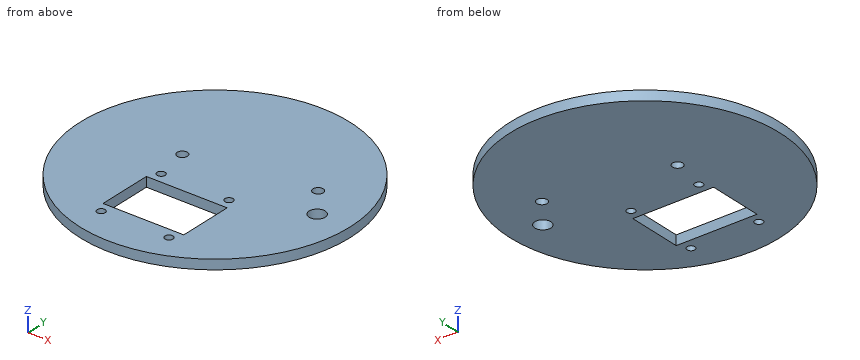
Autodesk Inventor part; units mm, degrees
ref_plane "YZ Plane" through (0, 0, 0) normal (1, 0, 0) x (0, 1, 0)
ref_plane "XZ Plane" through (0, 0, 0) normal (0, 1, 0) x (-1, 0, 0)
ref_plane "XY Plane" through (0, 0, 0) normal (0, 0, 1) x (1, 0, 0)
sketch "Эскиз3" plane through (0, 0, 0) normal (0, 0, 1) x (1, 0, 0)
  circle A0 centre (0, 0) radius 41.5
  line L0 (12.5, -11.0597) -> (-12.5, -11.0597)
  line L1 (-12.5, -11.0597) -> (-12.5, -28.0597)
  line L2 (-12.5, -11.0597) -> (12.5, -11.0597)
  line L3 (12.5, -11.0597) -> (12.5, -28.0597)
  line L4 (12.5, -28.0597) -> (-12.5, -28.0597)
  line L5 (-12.5, -28.0597) -> (-12.5, -11.0597)
  dimension "d9" = 83
  dimension "d10" = 25
  dimension "d11" = 17
  dimension "d13" = 25
  dimension "d14" = 17
  dimension "d15" = 12.5
extrude "Выдавливание3" add sketch "Эскиз3" along normal blind 3
sketch "Эскиз4" plane through (0, 0, 3) normal (0, 0, 1) x (1, 0, 0)
  arc A0 (5.7629, -8.6636) -> (-4.709, -8.7124) centre (0.4132, 15.7598) ccw
  circle A1 centre (0.4132, 15.7598) radius 1.5338
  point P0 (0, 0)
extrude "Выдавливание4" cut sketch "Эскиз4" against normal blind 3
sketch "Эскиз5" plane through (0, 0, 3) normal (0, 0, 1) x (1, 0, 0)
  line L0 (-51.8221, -46.0116) -> (-45.155, -49.3714)
  circle A0 centre (31.5626, 0.0623) radius 2.5
  point P0 (0, 0)
  dimension "d20" = 5
extrude "Выдавливание5" cut sketch "Эскиз5" against normal blind 3
sketch "Эскиз6" plane through (0, 0, 3) normal (0, 0, 1) x (1, 0, 0)
  circle A0 centre (0.4132, 15.7598) radius 1.5338
  point P0 (0, 0)
extrude "Выдавливание6" add sketch "Эскиз6" against normal blind 3
sketch "Эскиз7" plane through (0, 0, 3) normal (0, 0, 1) x (1, 0, 0)
  circle A0 centre (10.5, -7.8097) radius 1.25
  circle A1 centre (-10.5, -7.8097) radius 1.25
  circle A2 centre (-10.5, -31.3097) radius 1.25
  circle A3 centre (10.5, -31.3097) radius 1.25
  point P0 (0, 0)
extrude "Выдавливание7" cut sketch "Эскиз7" against normal blind 3
sketch "Эскиз13" plane through (0, 0, 3) normal (0, 0, 1) x (1, 0, 0)
  circle A0 centre (0, 0) radius 41.5
  circle A1 centre (0, 0) radius 41.7806
  point P0 (-26.934, 31.9403)
extrude "Выдавливание12" add sketch "Эскиз13" against normal blind 3
sketch "Эскиз14" plane through (0, 0, 0) normal (0, 0, -1) x (-1, 0, 0)
  circle A0 centre (-24.602, 9.2303) radius 1.6
  circle A1 centre (12.434, 2.9402) radius 1.6
  point P0 (0, 0)
extrude "Выдавливание13" cut sketch "Эскиз14" against normal blind 3
equation "\"d13\" = d10"
equation "\"d14\" = d11"
properties part number "top"
Model file for the job. Use its own axes, mm. Give positions to 0.01 mm unless a question says otherwise; leave off trailing zeros. Loops run counter-clockwise (first coordinate to the right, second up) from the corner with the lowest first, then second, coordinate; pieces in that order, holes last.
Item 1: Slice it at B-B (x = 10.5). Write the cut outline in (y, z), plus the area to 3 significant figures.
Check values:
outline: (-40.44, 0) - (-32.56, 0) - (-32.56, 3) - (-40.44, 3) - close; (-30.06, 0) - (-28.06, 0) - (-28.06, 3) - (-30.06, 3) - close; (-11.06, 0) - (-9.06, 0) - (-9.06, 3) - (-11.06, 3) - close; (-6.56, 0) - (40.44, 0) - (40.44, 3) - (-6.56, 3) - close
area: 177 mm2
Item 2: Slice it at D-D (x = 24.5). Write the cut outline in (y, z).
Check values:
outline: (-33.84, 0) - (7.63, 0) - (7.63, 3) - (-33.84, 3) - close; (10.83, 0) - (33.84, 0) - (33.84, 3) - (10.83, 3) - close
Item 3: Slice it at A-A (x = 0). Write the cut outline in (y, z), plus the area to 3 significant figures.
Check values:
outline: (-41.78, 0) - (-28.06, 0) - (-28.06, 3) - (-41.78, 3) - close; (-11.06, 0) - (41.78, 0) - (41.78, 3) - (-11.06, 3) - close
area: 200 mm2
Item 4: Drop flat-ended pins along their axis: P1, Ø1.5, axis at x = 28, z = 2, coming from the -Y side; P2, Ø1.5, axis at x = -5, z = 1.5, coming from the +Y side; P3, Ø1.5, axis at x = 2.5, z = 1.5, coming from the -Y side. Give the stop position or say it passes through.
Check values:
P1: stops at y = -31.67
P2: stops at y = 41.56
P3: stops at y = -41.74
Item 5: Slice it at C-C (z = 2.4). Give the number of separate pieces and of enclosed holes in the cut face, plus the area to 3 significant figures.
Check values:
separate pieces: 1
enclosed holes: 8
area: 5,000 mm2
Item 6: Drill centre lines: line 1 along Y through (x, z) = (10.5, 2); line 2 along Y through (x, z) = (10, 2.8); line 3 along X through (y, z) = (-1, 1.35). Where is each one in solid material? Low to high.
Check values:
line 1: y = -40.44 to -32.56, -30.06 to -28.06, -11.06 to -9.06, -6.56 to 40.44
line 2: y = -40.57 to -32.46, -30.16 to -28.06, -11.06 to -8.96, -6.66 to 40.57
line 3: x = -41.77 to 29.3, 33.83 to 41.77
